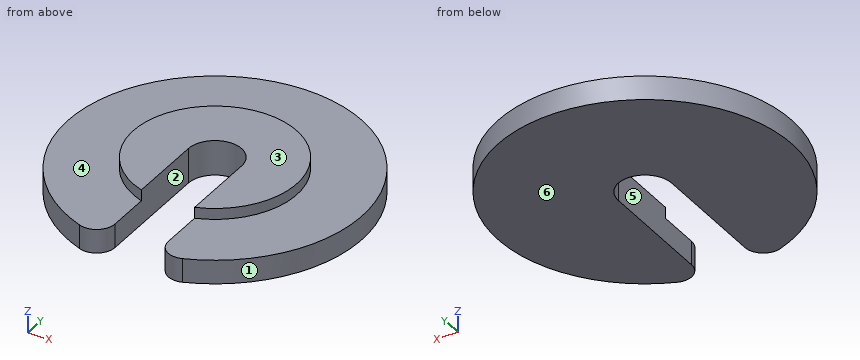
from build123d import *

# Parameters (mm, degrees)
F1_DEPTH = 1.9
F2_R     = 8
F2_R_2   = 4.45
F3_DEPTH = 0.6


with BuildPart() as f1:
    # F0 (on Top) → F1 (new body)
    with BuildSketch(Plane.XY):
        with BuildLine():
            ThreePointArc((-1.45, 0), (0, 1.45), (1.45, 0))
            Line((1.45, 0), (1.45, -6.5572478983))
            ThreePointArc((1.45, -6.5572478983), (1.8799122875, -7.3788317346), (2.8, -7.4939975981))
            ThreePointArc((2.8, -7.4939975981), (0, 8), (-2.8, -7.4939975981))
            ThreePointArc((-2.8, -7.4939975981), (-1.8799122875, -7.3788317346), (-1.45, -6.5572478983))
            Line((-1.45, -6.5572478983), (-1.45, 0))
        make_face()
    extrude(amount=F1_DEPTH)

    # F2 (on face) → F3 (cut)
    with BuildSketch(Plane.XY.offset(1.9)):
        Circle(F2_R)
        Circle(F2_R_2, mode=Mode.SUBTRACT)
    extrude(amount=-F3_DEPTH, mode=Mode.SUBTRACT)


solid = f1.part
Can you work these out from the model? Positions are in its coordinate system, mm. Face numbers are marked on the shaded views. A direction names the side the tool comes from. Give positions to 0.01 mm unless a question says otherwise; leave off trailing zeros. Write each loop counter-clockwise with the first axis right and the second up, starting at its lowest first coordinate (ties: lowest second). Pieces come first, ordered by that corner, then holes. Notation, with made-up numbers: (0, 27) -> (51, 27) arc R13 ccw to (51, 45) -> close; hole circle Ø8 at (59, 75). An arc over 180 degrees is marked (long way). Answer as a JSON object with one key per item and string values. Group by question number.
Item 1: I'm going to push flat-ended pins straight in: P1, Ø1, axis at y = -2, z = 0.5, coming from the +X side; P2, Ø1, axis at y = -3, z = 1.5, coming from the -X side; P3, Ø2, axis at x = 0.5, y = 2.5, coming from the -Z side. Where does each tip first touch, or does it pass through?
Item 2: Suppose I cut it at D-D (x = -3.75). Please give me the cut outline in (y, z).
Item 3: For the marked faces 4, 5 and 6, which set-ups out of +Z, -Z, +X, -X, +Y, -Y let a thin tool reach every point of the face, with its end or its side?
Item 4: Suppose I cut it at A-A (y = -1.5). Please give me the cut outline in (x, z), plus the area to 3 significant figures.
Item 5: Suppose I cut it at B-B (x = 0). Please give me the cut outline in (y, z), plus the area to 3 significant figures.
Item 6: Suppose I cut it at C-C (z = 0.55). Please give me the cut outline in (x, y), plus the area to 3 significant figures.
Item 7: Please list where these lines run through material, in increasing order: line 1 (Z direction, x = 1, y = 4.5); line 2 (X direction, y = -1.75, z = 1.4); line 3 (X direction, y = -4.25, z = 0.9). Write a range as [from, to].
Item 8: We'd pull the mould along X, two halves only. Please class the marked faces 1, 2 and 3: +X half, -X half, draft (parallel to the pull), parting line (faces both ways), or undercut.
Findings:
{
 "1": {"P1": "stops at x = 7.86", "P2": "stops at x = -7.59", "P3": "stops at z = 0"},
 "2": {"outline": "(-7.07, 0) -> (7.07, 0) -> (7.07, 1.3) -> (2.4, 1.3) -> (2.4, 1.9) -> (-2.4, 1.9) -> (-2.4, 1.3) -> (-7.07, 1.3) -> close"},
 "3": {"face 4": "+Z", "face 5": "+Z, -Z, -Y", "face 6": "-Z, +X, -X, +Y, -Y"},
 "4": {"outline": "(-7.86, 0) -> (-1.45, 0) -> (-1.45, 1.9) -> (-4.19, 1.9) -> (-4.19, 1.3) -> (-7.86, 1.3) -> close; (1.45, 0) -> (7.86, 0) -> (7.86, 1.3) -> (4.19, 1.3) -> (4.19, 1.9) -> (1.45, 1.9) -> close", "area": "19.9 mm²"},
 "5": {"outline": "(1.45, 0) -> (8, 0) -> (8, 1.3) -> (4.45, 1.3) -> (4.45, 1.9) -> (1.45, 1.9) -> close", "area": "10.3 mm²"},
 "6": {"outline": "(-2.8, -7.49) arc R1 ccw to (-1.45, -6.56) -> (-1.45, 0) arc R1.45 cw to (1.45, 0) -> (1.45, -6.56) arc R1 ccw to (2.8, -7.49) arc R8 ccw (long way) to start", "area": "174 mm²"},
 "7": {"line 1": "z = [0, 1.3]", "line 2": "x = [-4.09, -1.45], [1.45, 4.09]", "line 3": "x = [-6.78, -1.45], [1.45, 6.78]"},
 "8": {"face 1": "parting line", "face 2": "undercut", "face 3": "draft"}
}
